The listing builds one solid part. Answer for the finished solid, in the listing's coordinates (mm). Face numbers are marked on the shaded views. A direction names the side the tool comes from. Round coordinates to 2 decimals unless told otherwise and drop trailing zeros. Write each loop counter-clockwise with the first axis right and the second up, starting at its lowest first coordinate (ties: lowest second). Pieces come first, ordered by that corner, then holes. Notation, with made-up numbers: (-38, 59.5) - (-30, 59.5) arc R25 ccw to (-30, 94.5) - close; hole circle Ø5 at (32.5, -29). An arc over 180 degrees is marked (long way). Answer in a Markdown table with one row per item.
from build123d import *

# Parameters (mm, degrees)
F1_DEPTH = 101.6
F2_R     = 6.35
F3_DEPTH = 25.4
F4_R     = 6.35
F5_DEPTH = 25.4
F6_W     = 1.778
F6_H     = 7.62
F7_DEPTH = 2.54


with BuildPart() as f1:
    # F0 (on Front) → F1 (new body)
    with BuildSketch(Plane.XZ):
        Polygon((62.0224951868, 69.85), (19.05, 69.85), (0, 50.8), (0, 0), (6.1424951868, 0), (6.1424951868, 50.8), (20.1124951868, 64.77), (60.7524951868, 64.77), (74.7224951868, 50.8), (74.7224951868, 0), (81.0724951868, 0), (81.0724951868, 50.8), align=None)
    extrude(amount=F1_DEPTH)

    # F2 (on face) → F3 (cut)
    with BuildSketch(Plane(origin=(65.9362475934, 0, 65.9362475934), x_dir=(0, 1, 0), z_dir=(0.7071067812, 0, 0.7071067812))):
        with Locations((-12.7, -7.9355024484)):
            Circle(F2_R)
        with Locations((-38.1, -7.9355024484)):
            Circle(F2_R)
        with Locations((-63.5, -7.9355024484)):
            Circle(F2_R)
        with Locations((-88.9, -7.9355024484)):
            Circle(F2_R)
    extrude(amount=-F3_DEPTH, mode=Mode.SUBTRACT)

    # F4 (on face) → F5 (cut)
    with BuildSketch(Plane(origin=(-25.4, 0, 25.4), x_dir=(0, -1, 0), z_dir=(-0.7071067812, 0, 0.7071067812))):
        with Locations((88.9, 49.3914086659)):
            Circle(F4_R)
        with Locations((63.5, 49.3914086659)):
            Circle(F4_R)
        with Locations((38.1, 49.3914086659)):
            Circle(F4_R)
        with Locations((12.7, 49.3914086659)):
            Circle(F4_R)
    extrude(amount=-F5_DEPTH, mode=Mode.SUBTRACT)

    # F6 (on face) → F7 (join)
    with BuildSketch(Plane(origin=(-22.3287524066, 0, 22.3287524066), x_dir=(0, 1, 0), z_dir=(0.7071067812, 0, -0.7071067812))):
        with Locations((-96.901, 50.1427062175)):
            Rectangle(F6_W, F6_H)
        with Locations((-81.153, 50.1427062175)):
            Rectangle(F6_W, F6_H)
        with Locations((-71.247, 50.1427062175)):
            Rectangle(F6_W, F6_H)
        with Locations((-55.499, 50.1427062175)):
            Rectangle(F6_W, F6_H)
        with Locations((-46.101, 50.1427062175)):
            Rectangle(F6_W, F6_H)
        with Locations((-30.353, 50.1427062175)):
            Rectangle(F6_W, F6_H)
        with Locations((-20.447, 50.1427062175)):
            Rectangle(F6_W, F6_H)
        with Locations((-4.699, 50.1427062175)):
            Rectangle(F6_W, F6_H)
    extrude(amount=F7_DEPTH)


solid = f1.part
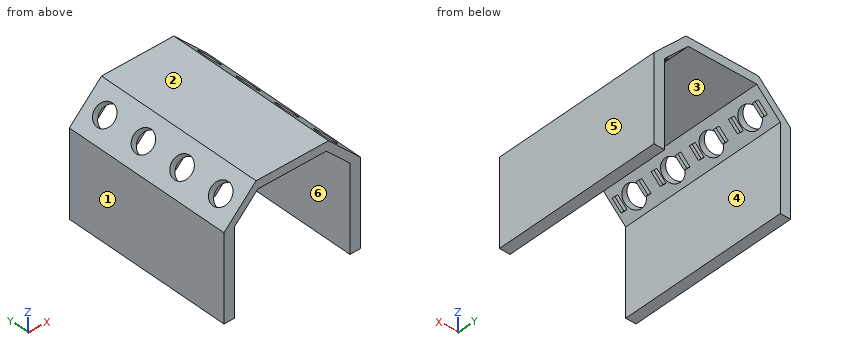
(1) Section A-A (z = 33) is taken. Give the vertices of the cut face in (x, y).
Checked values:
| item | result |
|---|---|
| outline | (0, -101.6) - (6.14, -101.6) - (6.14, 0) - (0, 0) - close; (74.72, -101.6) - (81.07, -101.6) - (81.07, 0) - (74.72, 0) - close |
(2) Flat-ended cylindrical pins translate along their axes: pin 1 (2 mm diameter, centred on x = 65, y = -49, fed in from -Z); pin 2 (3.5 mm diameter, centred on x = 15, z = 55.5, fed in from +Y); pin 3 (12 mm diameter, centred on x = 39.5, y = -41.5, fed in from -Z). Find the tip coordinate at first contact, or state that the pin passes through.
Checked values:
| item | result |
|---|---|
| pin 1 | stops at z = 59.52 |
| pin 2 | stops at y = -3.81 |
| pin 3 | stops at z = 64.77 |
(3) For a pull along X with two mould halves and no side action, classify the marked faces 1, 2, 3 and 4 as pulls with the +X half, pulls with the -X half, needs draft (parallel to the pull), parting line crosses it, or undercut.
Checked values:
| item | result |
|---|---|
| face 1 | pulls with the -X half |
| face 2 | needs draft |
| face 3 | undercut |
| face 4 | undercut |
(4) Section D-D (x = 39.5) is taken. Give the vertices of the cut face in (y, z), and give its area (3 significant figures).
Checked values:
| item | result |
|---|---|
| outline | (-101.6, 64.77) - (0, 64.77) - (0, 69.85) - (-101.6, 69.85) - close |
| area | 516 mm2 |
(5) Section C-C (y = -17.5) is taken. Give the vertices of the cut face in (x, z).
Checked values:
| item | result |
|---|---|
| outline | (0, 0) - (6.14, 0) - (6.14, 50.8) - (9.66, 54.31) - (6.59, 57.39) - (0, 50.8) - close; (12.46, 63.26) - (15.54, 60.19) - (20.11, 64.77) - (60.75, 64.77) - (65.43, 60.09) - (68.61, 63.26) - (62.02, 69.85) - (19.05, 69.85) - close; (71.31, 54.21) - (74.72, 50.8) - (74.72, 0) - (81.07, 0) - (81.07, 50.8) - (74.49, 57.39) - close |
(6) Section B-B (y = -61) is taken. State how many separate pieces and enclosed holes the cut face has, and give its area (3 significant figures).
Checked values:
| item | result |
|---|---|
| separate pieces | 3 |
| enclosed holes | 0 |
| area | 950 mm2 |
(7) Find the intervals of material crossed by line 1 (X direction, y = -66.5, z = 25); line 2 (Z direction, x = 23, y = -14); line 3 (X direction, y = -28.5, z = 58), in increasing order.
Checked values:
| item | result |
|---|---|
| line 1 | x = 0 to 6.14, 74.72 to 81.07 |
| line 2 | z = 64.77 to 69.85 |
| line 3 | x = 7.2 to 13.34, 67.52 to 73.87 |
(8) For the marked faces 5 and 6, determine the directions among +Z, -Z, +X, -X, +Y, -Y from which every point of the face is accessible in a straight line to the end or side of a thin tool.
Checked values:
| item | result |
|---|---|
| face 5 | +Z, -Z, +X, +Y, -Y |
| face 6 | -Z, +Y, -Y |
